The model under review builds one solid part; all positions refer to its coordinate system, in mm. Coordinates: 2 decimals unless noted, no trailing zeros. Write each loop counter-clockwise with the first axis right and the second up, starting at its lowest first coordinate (ties: lowest second). Pieces come first, ordered by that corner, then holes. Notation, with made-up numbers: (53, -31.5) -> (99, -31.5) arc R13 cw to (99, -25.5) -> close; hole circle Ø8 at (88, -34). An arc over 180 degrees is marked (long way). Write each question's results on one line, items separated by ' | '.
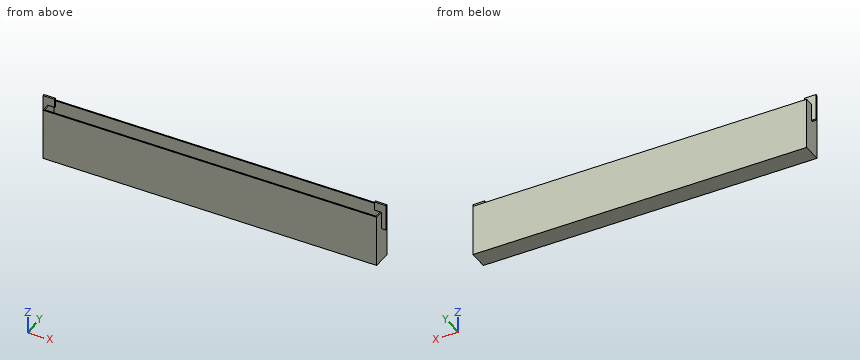
```python
from build123d import *

# Parameters (mm, degrees)
F0_W      = 570
F0_H      = 32
F1_DEPTH  = 89
F2_W      = 3
F2_H      = 30
F3_DEPTH  = 8
F4_W      = 8
F4_H      = 3
F5_DEPTH  = 15
F6_W      = 566
F6_H      = 28
F7_DEPTH  = 87
F8_W      = 3
F8_H      = 15
F9_DEPTH  = 12
F10_W     = 3
F10_H     = 30
F10_H_2   = 15
F11_DEPTH = 8
F12_W     = 3
F12_H     = 15
F13_DEPTH = 12


with BuildPart() as f1:
    # F0 (on Top) → F1 (new body)
    with BuildSketch(Plane.XY):
        Rectangle(F0_W, F0_H)
    extrude(amount=F1_DEPTH)

    # F2 (on face) → F3 (join)
    with BuildSketch(Plane(origin=(-285, 0, 0), x_dir=(0, -1, 0), z_dir=(-1, 0, 0))):
        with Locations((0, 74)):
            Rectangle(F2_W, F2_H)
    extrude(amount=F3_DEPTH)

    # F4 (on face) → F5 (join)
    with BuildSketch(Plane.XY.offset(89)):
        with Locations((-289, 0)):
            Rectangle(F4_W, F4_H)
    extrude(amount=F5_DEPTH)

    # F6 (on face) → F7 (cut)
    with BuildSketch(Plane.XY.offset(89)):
        Rectangle(F6_W, F6_H)
    extrude(amount=-F7_DEPTH, mode=Mode.SUBTRACT)

    # F8 (on face) → F9 (join)
    with BuildSketch(Plane(origin=(285, 0, 0), x_dir=(0, -1, 0), z_dir=(-1, 0, 0))):
        with Locations((0, 96.5)):
            Rectangle(F8_W, F8_H)
    extrude(amount=F9_DEPTH)

    # F10 (on face) → F11 (join)
    with BuildSketch(Plane.YZ.offset(285)):
        with Locations((0, 74)):
            Rectangle(F10_W, F10_H)
        with Locations((0, 96.5)):
            Rectangle(F10_W, F10_H_2)
    extrude(amount=F11_DEPTH)

    # F12 (on face) → F13 (join)
    with BuildSketch(Plane.YZ.offset(-285)):
        with Locations((0, 96.5)):
            Rectangle(F12_W, F12_H)
    extrude(amount=F13_DEPTH)


solid = f1.part
```
Q1. Add section B-B (z = 49). Write out the cut boundary in (x, y).
Solution:
outline: (-285, -16) -> (285, -16) -> (285, 16) -> (-285, 16) -> close; hole (-283, -14) -> (283, -14) -> (283, 14) -> (-283, 14) -> close
Q2. Add section A-A (z = 94). Write out the cut boundary in (x, y).
Solution:
outline: (-293, -1.5) -> (-273, -1.5) -> (-273, 1.5) -> (-293, 1.5) -> close; (273, -1.5) -> (293, -1.5) -> (293, 1.5) -> (273, 1.5) -> close
Q3. Add section D-D (y = -7). Write out the cut boundary in (x, z), plus the area to 3 significant figures.
Solution:
outline: (-285, 0) -> (285, 0) -> (285, 89) -> (283, 89) -> (283, 2) -> (-283, 2) -> (-283, 89) -> (-285, 89) -> close | area: 1,490 mm²
Q4. For line 1 (Y direction, x = 3.5, z = 87); line 2 (X direction, y = 4, z = 9.5); line 3 (Z direction, x = 150.5, y = 7), list the stretches that pass through material, from the lowest coordinate up. Write a range as from..to.
Solution:
line 1: -16..-14, 14..16 | line 2: -285..-283, 283..285 | line 3: 0..2
Q5. Add section C-C (x = 243.5). Write out the cut boundary in (y, z).
Solution:
outline: (-16, 0) -> (16, 0) -> (16, 89) -> (14, 89) -> (14, 2) -> (-14, 2) -> (-14, 89) -> (-16, 89) -> close
Q6. Clearance check with flat-ended pins moving along their axes: P1, Ø9.5, axis at y = -6.5, z = 53.5, coming from the -X side; P2, Ø14, axis at x = -26, y = -4, coming from the +Z side; P3, Ø0.9, axis at x = 287, y = 0, coming from the -Z side. State where each tip first meets the part, or that it passes through.
Solution:
P1: x = -285 | P2: z = 2 | P3: z = 59
